from build123d import *

# Parameters (mm, degrees)
SKETCH_1_R          = 80
EXTRUDE_1_DEPTH     = 302
SKETCH_2_R          = 265
EXTRUDE_2_DEPTH     = 14
SKETCH_3_R          = 265
EXTRUDE_3_DEPTH     = 14
SKETCH_4_R          = 40
CUT_EXTRUDE_1_DEPTH = 331


with BuildPart() as part:
    # Эскиз1 → Бобышка-Вытянуть1 (new body)
    with BuildSketch(Plane.XY):
        Circle(SKETCH_1_R)
    extrude(amount=EXTRUDE_1_DEPTH)

    # Эскиз2 → Бобышка-Вытянуть2 (add)
    with BuildSketch(Plane(origin=(0, 0, 0), x_dir=(-1, 0, 0), z_dir=(0, 0, -1))):
        Circle(SKETCH_2_R)
    extrude(amount=EXTRUDE_2_DEPTH)

    # Эскиз3 → Бобышка-Вытянуть3 (add)
    with BuildSketch(Plane.XY.offset(302)):
        Circle(SKETCH_3_R)
    extrude(amount=EXTRUDE_3_DEPTH)

    # Эскиз4 → Вырез-Вытянуть1 (cut, through all)
    with BuildSketch(Plane(origin=(0, 0, -14), x_dir=(-1, 0, 0), z_dir=(0, 0, -1))):
        Circle(SKETCH_4_R)
    extrude(amount=-CUT_EXTRUDE_1_DEPTH, mode=Mode.SUBTRACT)


solid = part.part
Design review of the part built by this model. Coordinates are the model's own, in mm. A direction names the side the tool comes from. Round coordinates to 2 decimals unless told otherwise and drop trailing zeros. Order: outer loops, then holes, each group sorted by start corner. A loop starts at its lowest first (then second) coordinate and runs counter-clockwise, first axis right, second up. Notation, with made-up numbers: M -6,21.25 L 9,21.25 A12 ccw 9,42.25 Z; hole C -38.75,-20.75 d9. An arc over 180 degrees is marked long. Answer as CSV lines item,"result". Start each with the question number.
1) Tool access review of faces 4 (the face through (-17.34, -78.1, 148.89)), 5 (the face through (-142.46, 223.45, -6.9)): name each direction out of +Z, -Z, +X, -X, +Y, -Y from which nothing blocks a thin tool from reaching the whole face with its end or side.
2) For pin 1 Ø12 at (y, z) = (-4, 174) entering from +X; pin 2 Ø12 at (x, z) = (64.5, 108) entering from +Y, all flat-tipped, find the tip position at first contact; note any pin that passes through.
3) Add section D-D (y = 230). Give the boundary of the cut face in (x, z), then the cut area to 3 significant figures.
4) Add section C-C (z = 13). Give the boundary of the cut face in (x, y), then the cut area to 3 significant figures.
5) The part is to be moulded in two halves that separate along X. For faces 1 (the face through (142.46, 223.45, 308.9)), 2 (the face through (8.67, -39.05, 148.69)), 3 (the face through (55, 4, 316)), say which applies: +X half, -X half, draft (parallel to the pull), parting line (faces both ways), or undercut.
6) Add section A-A (x = 0). Give the boundary of the cut face in (y, z), then the cut area to 3 significant figures.
7) Wall thickness on line 1 along Y through (x, z) = (0, 129); line 2 along Z through (x, y) = (58, 148.5); line 3 along X through (y, z) = (-5, 12): over which ranges is each line inside the solid? List them lowest first. Write a range as [from, to].
Resolved:
1,face 4,"none"
1,face 5,"+Z, -Z"
2,pin 1,"x = 80"
2,pin 2,"y = 54.57"
3,outline,"M -131.62,-14 L 131.62,-14 L 131.62,0 L -131.62,0 Z; M -131.62,302 L 131.62,302 L 131.62,316 L -131.62,316 Z"
3,area,"7,370 mm^2"
4,outline,"C 0,0 d160; hole C 0,0 d80"
4,area,"15,100 mm^2"
5,face 1,"parting line"
5,face 2,"undercut"
5,face 3,"draft"
6,outline,"M -265,-14 L -40,-14 L -40,316 L -265,316 L -265,302 L -80,302 L -80,0 L -265,0 Z; M 40,-14 L 265,-14 L 265,0 L 80,0 L 80,302 L 265,302 L 265,316 L 40,316 Z"
6,area,"36,800 mm^2"
7,line 1,"[-80, -40], [40, 80]"
7,line 2,"[-14, 0], [302, 316]"
7,line 3,"[-79.84, -39.69], [39.69, 79.84]"
